Geometry check sheet. Reference: drawing and pictorial views, mm from the part's lowest x, y, z. A direction names the side the tool comes from. Give positions to 0.01 mm unless a question says otherwise; leave off trailing zeros. Write each loop counter-clockwise with the first axis right and the second up, starting at its lowest first coordinate (ties: lowest second). Pieces come first, ordered by that corner, then holes.
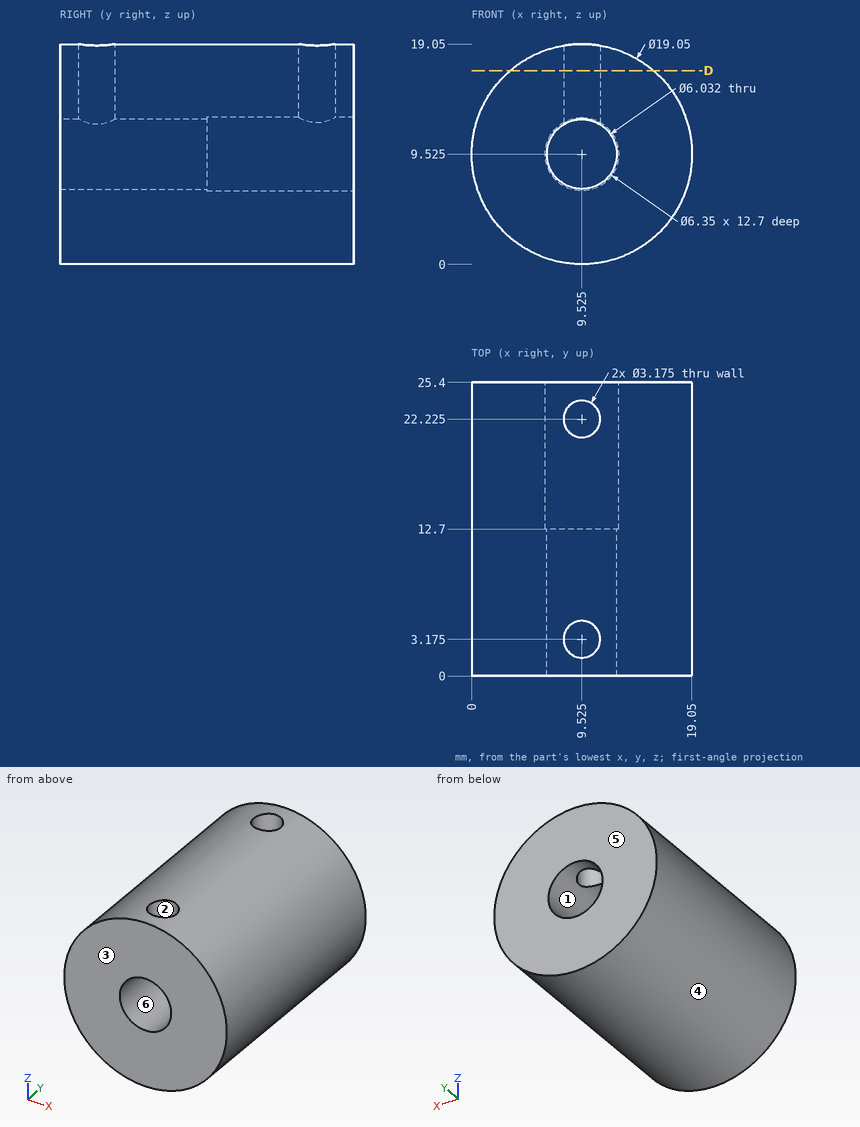
Item 1: Set-up check for the marked faces 1, 2 and 3: record each of +Z, -Z, +X, -X, +Y, -Y from which the full face is reachable in a straight line by a thin tool's end or side.
Answer key:
face 1: +Y
face 2: +Z
face 3: +Z, -Z, +X, -X, -Y
Item 2: Sectioned sample at D-D on z = 16.75. Record the cut outline in (x, y) (1 decimal).
Answer key:
outline: (3.3, 0) - (15.7, 0) - (15.7, 25.4) - (3.3, 25.4) - close; hole circle Ø3.2 at (9.5, 3.2); hole circle Ø3.2 at (9.5, 22.2)
Item 3: Depth check by flat-ended pin: pin 1 (1.5 mm diameter, centred on x = 16.5, y = 11.5, fed in from +Z) (1 decimal); pin 2 (6 mm diameter, centred on x = 12, y = 19, fed in from +Z); pin 3 (4 mm diameter, centred on x = 9.525, z = 9.525, fed in from -Y); pin 4 (6 mm diameter, centred on x = 14.5, y = 5, fed in from -Z). Enter the tip coordinate at first touch or a pass-through.
Answer key:
pin 1: stops at z = 16.7
pin 2: stops at z = 19.05
pin 3: passes through
pin 4: stops at z = 0.21
Item 4: Scan lines: line 1 along Y through (x, z) = (9.5, 13.75); line 2 along Y through (x, z) = (9.75, 17); line 3 along X through (y, z) = (23.25, 13) (1 decimal). Record each from-to range of solid material in increasing order.
Answer key:
line 1: y = 0 to 1.59, 4.76 to 20.64, 23.81 to 25.4
line 2: y = 0 to 1.6, 4.75 to 20.65, 23.8 to 25.4
line 3: x = 0.7 to 8.3, 10.7 to 18.4
Item 5: Release check for a two-part mould opening along X. For the marked faces 4, 5 and 6 record: released by +X, released by -X, zero draft, split by the parting line, or undercut.
Answer key:
face 4: split by the parting line
face 5: zero draft
face 6: undercut
